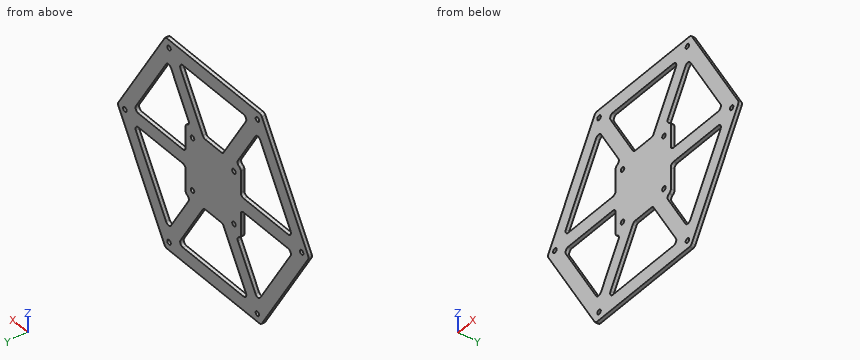
```python
from build123d import *

# Parameters (mm, degrees)
SKETCH1_R           = 3.2
BOSS_EXTRUDE1_DEPTH = 10
SKETCH2_W           = 100
SKETCH2_H           = 100
BOSS_EXTRUDE2_DEPTH = 10
FILLET1_R           = 5
FILLET2_R           = 5
SKETCH3_R           = 3.2
CUT_EXTRUDE2_DEPTH  = 10
CUT_EXTRUDE3_START  = -5
CUT_EXTRUDE3_DEPTH  = 5


with BuildPart() as part:
    # Sketch1 → Boss-Extrude1 (new body)
    with BuildSketch(Plane(origin=(0, 0, 0), x_dir=(1, 0, 0), z_dir=(0, 1, 0))):
        with BuildLine():
            ThreePointArc((171.761705084, -2.5), (172.431578065, 0), (171.761705084, 2.5))
            Line((171.761705084, 2.5), (88.045916051, 147.5))
            ThreePointArc((88.045916051, 147.5), (86.215789032, 149.330127019), (83.715789032, 150))
            Line((83.715789032, 150), (-83.715789032, 150))
            ThreePointArc((-83.715789032, 150), (-86.215789032, 149.330127019), (-88.045916051, 147.5))
            Line((-88.045916051, 147.5), (-171.761705084, 2.5))
            ThreePointArc((-171.761705084, 2.5), (-172.431578065, 0), (-171.761705084, -2.5))
            Line((-171.761705084, -2.5), (-88.045916051, -147.5))
            ThreePointArc((-88.045916051, -147.5), (-86.215789032, -149.330127019), (-83.715789032, -150))
            Line((-83.715789032, -150), (83.715789032, -150))
            ThreePointArc((83.715789032, -150), (86.215789032, -149.330127019), (88.045916051, -147.5))
            Line((88.045916051, -147.5), (171.761705084, -2.5))
        make_face()
        with Locations(Location((-80, -138.564064606, 0), (0, 0, 270))):
            Circle(SKETCH1_R, mode=Mode.SUBTRACT)
        with Locations(Location((80, -138.564064606, 0), (0, 0, 270))):
            Circle(SKETCH1_R, mode=Mode.SUBTRACT)
        with Locations(Location((-160, 0, 0), (0, 0, 270))):
            Circle(SKETCH1_R, mode=Mode.SUBTRACT)
        with Locations(Location((-80, 138.564064606, 0), (0, 0, 270))):
            Circle(SKETCH1_R, mode=Mode.SUBTRACT)
        with BuildLine():
            ThreePointArc((-85.159164705, 112.5), (-80.829037687, 115), (-76.498910668, 112.5))
            Line((-76.498910668, 112.5), (-40.414518843, 50))
            Line((-40.414518843, 50), (-17.320508076, 50))
            Line((-17.320508076, 50), (-59.178402592, 122.5))
            ThreePointArc((-59.178402592, 122.5), (-59.178402592, 127.5), (-54.848275573, 130))
            Line((-54.848275573, 130), (54.848275573, 130))
            ThreePointArc((54.848275573, 130), (59.178402592, 127.5), (59.178402592, 122.5))
            Line((59.178402592, 122.5), (17.320508076, 50))
            Line((17.320508076, 50), (40.414518843, 50))
            Line((40.414518843, 50), (76.498910668, 112.5))
            ThreePointArc((76.498910668, 112.5), (80.829037687, 115), (85.159164705, 112.5))
            Line((85.159164705, 112.5), (140.007440278, 17.5))
            ThreePointArc((140.007440278, 17.5), (140.007440278, 12.5), (135.67731326, 10))
            Line((135.67731326, 10), (50, 10))
            Line((50, 10), (50, -10))
            Line((50, -10), (135.67731326, -10))
            ThreePointArc((135.67731326, -10), (140.007440278, -12.5), (140.007440278, -17.5))
            Line((140.007440278, -17.5), (85.159164705, -112.5))
            ThreePointArc((85.159164705, -112.5), (80.829037687, -115), (76.498910668, -112.5))
            Line((76.498910668, -112.5), (40.414518843, -50))
            Line((40.414518843, -50), (17.320508076, -50))
            Line((17.320508076, -50), (59.178402592, -122.5))
            ThreePointArc((59.178402592, -122.5), (59.178402592, -127.5), (54.848275573, -130))
            Line((54.848275573, -130), (-54.848275573, -130))
            ThreePointArc((-54.848275573, -130), (-59.178402592, -127.5), (-59.178402592, -122.5))
            Line((-59.178402592, -122.5), (-17.320508076, -50))
            Line((-17.320508076, -50), (-40.414518843, -50))
            Line((-40.414518843, -50), (-76.498910668, -112.5))
            ThreePointArc((-76.498910668, -112.5), (-80.829037687, -115), (-85.159164705, -112.5))
            Line((-85.159164705, -112.5), (-140.007440278, -17.5))
            ThreePointArc((-140.007440278, -17.5), (-140.007440278, -12.5), (-135.67731326, -10))
            Line((-135.67731326, -10), (-50, -10))
            Line((-50, -10), (-50, 10))
            Line((-50, 10), (-135.67731326, 10))
            ThreePointArc((-135.67731326, 10), (-140.007440278, 12.5), (-140.007440278, 17.5))
            Line((-140.007440278, 17.5), (-85.159164705, 112.5))
        make_face(mode=Mode.SUBTRACT)
        with Locations(Location((160, 0, 0), (0, 0, 270))):
            Circle(SKETCH1_R, mode=Mode.SUBTRACT)
        with Locations(Location((80, 138.564064606, 0), (0, 0, 270))):
            Circle(SKETCH1_R, mode=Mode.SUBTRACT)
    extrude(amount=BOSS_EXTRUDE1_DEPTH)

    # Sketch2 → Boss-Extrude2 (add)
    with BuildSketch(Plane(origin=(0, 0, 0), x_dir=(1, 0, 0), z_dir=(0, 1, 0))):
        Rectangle(SKETCH2_W, SKETCH2_H)
    extrude(amount=BOSS_EXTRUDE2_DEPTH)

    # Fillet1
    fillet1_edges = [part.edges().sort_by_distance(p)[0] for p in [
        (-50, 5, -10),
        (-50, 5, 10),
        (-40.414518843, 5, 50),
        (-17.320508076, 5, 50),
        (17.320508076, 5, 50),
        (40.414518843, 5, 50),
        (50, 5, 10),
        (50, 5, -10),
        (40.414518843, 5, -50),
        (17.320508076, 5, -50),
        (-17.320508076, 5, -50),
        (-40.414518843, 5, -50),
    ]]
    fillet(fillet1_edges, radius=FILLET1_R)

    # Fillet2
    fillet2_edges = [part.edges().sort_by_distance(p)[0] for p in [
        (-50, 5, -50),
        (-50, 5, 50),
        (50, 5, 50),
        (50, 5, -50),
    ]]
    fillet(fillet2_edges, radius=FILLET2_R)

    # Sketch3 → Cut-Extrude2 (cut)
    with BuildSketch(Plane(origin=(0, 10, 0), x_dir=(1, 0, 0), z_dir=(0, 1, 0))):
        with Locations(Location((-37.5, 37.5, 0), (0, 0, 270))):
            Circle(SKETCH3_R)
        with Locations(Location((37.5, 37.5, 0), (0, 0, 270))):
            Circle(SKETCH3_R)
        with Locations(Location((37.5, -37.5, 0), (0, 0, 270))):
            Circle(SKETCH3_R)
        with Locations(Location((-37.5, -37.5, 0), (0, 0, 270))):
            Circle(SKETCH3_R)
    extrude(amount=-CUT_EXTRUDE2_DEPTH, mode=Mode.SUBTRACT)

    # Sketch6 → Cut-Extrude3 (cut)
    with BuildSketch(Plane(origin=(0, 10, 0), x_dir=(1, 0, 0), z_dir=(0, 1, 0)).offset(CUT_EXTRUDE3_START)):
        with BuildLine():
            Line((88.045916051, 147.5), (171.761705084, 2.5))
            ThreePointArc((171.761705084, 2.5), (172.431578065, 0), (171.761705084, -2.5))
            Line((171.761705084, -2.5), (88.045916051, -147.5))
            ThreePointArc((88.045916051, -147.5), (86.215789032, -149.330127019), (83.715789032, -150))
            Line((83.715789032, -150), (-83.715789032, -150))
            ThreePointArc((-83.715789032, -150), (-86.215789032, -149.330127019), (-88.045916051, -147.5))
            Line((-88.045916051, -147.5), (-171.761705084, -2.5))
            ThreePointArc((-171.761705084, -2.5), (-172.431578065, 0), (-171.761705084, 2.5))
            Line((-171.761705084, 2.5), (-88.045916051, 147.5))
            ThreePointArc((-88.045916051, 147.5), (-86.215789032, 149.330127019), (-83.715789032, 150))
            Line((-83.715789032, 150), (83.715789032, 150))
            ThreePointArc((83.715789032, 150), (86.215789032, 149.330127019), (88.045916051, 147.5))
        make_face()
    extrude(amount=CUT_EXTRUDE3_DEPTH, mode=Mode.SUBTRACT)


solid = part.part
```
Build history of the part. All positions in model axes, mm. Round coordinates to 2 decimals unless told otherwise and drop trailing zeros. Loops run counter-clockwise (first coordinate to the right, second up) from the corner with the lowest first, then second, coordinate; pieces in that order, holes last.
Item 1: Drill centre lines: line 1 along Z through (x, y) = (-80, 1.1); line 2 along Z through (x, y) = (10.5, 3.6); line 3 along X through (y, z) = (2.8, 69.5). Where is each one in solid material? Low to high.
Item 2: Saw through at C-C (y = 2.7). State how many separate pieces and enclosed holes the cut face has, then the cut area to 3 significant figures.
Item 3: Saw through at A-A (z = -73). List the corners of the cut face in (x, y).
Item 4: Pin check, flat tips, straight feed: P1, Ø2.5, axis at y = 2.5, z = -28.5, coming from the +X side; P2, Ø1.5, axis at y = 3, z = 34.5, coming from the +X side; P3, Ø2, axis at y = 3.5, z = -15.5, coming from the +X side. Stop position of each tip, or through.
Item 5: Saw through at B-B (x = 122.5). List the corners of the cut face in (y, z).
Worked answers:
1. line 1: z = -150 to -141.76, -135.36 to -114.93, -10 to 10, 114.93 to 135.36, 141.76 to 150
1. line 2: z = -150 to -130, -50 to 50, 130 to 150
1. line 3: x = -133.08 to -109.99, -51.67 to -28.58, 28.58 to 51.67, 109.99 to 133.08
2. separate pieces: 1
2. enclosed holes: 16
2. area: 40,400 mm2
3. outline: (-131.06, 0) - (-107.96, 0) - (-107.96, 5) - (-131.06, 5) - close; (-53.69, 0) - (-30.6, 0) - (-30.6, 5) - (-53.69, 5) - close; (30.6, 0) - (53.69, 0) - (53.69, 5) - (30.6, 5) - close; (107.96, 0) - (131.06, 0) - (131.06, 5) - (107.96, 5) - close
4. P1: stops at x = 157.47
4. P2: stops at x = 153.72
4. P3: stops at x = 164.83
5. outline: (0, -87.82) - (5, -87.82) - (5, -47.82) - (0, -47.82) - close; (0, -10) - (5, -10) - (5, 10) - (0, 10) - close; (0, 47.82) - (5, 47.82) - (5, 87.82) - (0, 87.82) - close
